Could you check a few things on this model? Use its own coordinates, in mm. Face numbers are marked on the shaded views. Coordinates: 2 decimals unless noted, no trailing zeros. Loops run counter-clockwise (first coordinate to the right, second up) from the corner with the lowest first, then second, coordinate; pieces in that order, holes last. Notation, with made-up numbers: (-18, -10) - (1, -10) arc R37 ccw to (1, 26) - close; hole circle Ø11 at (20, 24.25). An arc over 180 degrees is marked (long way). Use CSV: the item, a comma, the result in double quotes.
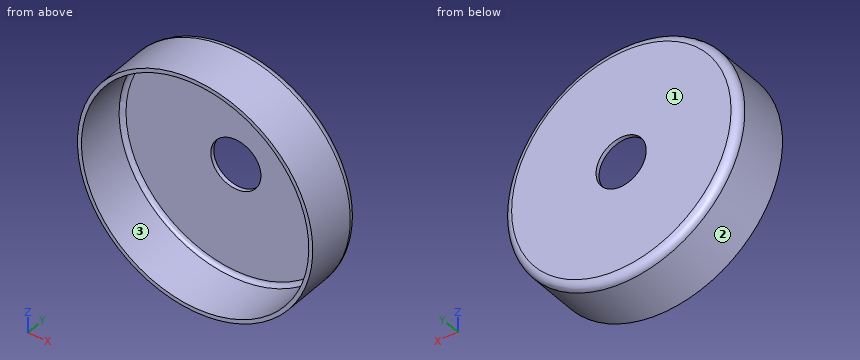
from build123d import *

# Parameters (mm, degrees)
SKETCH1_W               = 141.4859375
SKETCH1_H               = 69.85
FILLET1_R               = 9.525
SHELL1_T                = -4.7625
SKETCH3_R               = 30.1625
CUT_EXTRUDE1_DEPTH      = 30.734
CUT_EXTRUDE1_DEPTH_BACK = 28.194


with BuildPart() as part:
    # Sketch1 → Revolve1 (revolve)
    with BuildSketch(Plane(origin=(0, 0, 0), x_dir=(0, 0, -1), z_dir=(1, 0, 0)), mode=Mode.PRIVATE) as revolve1_sk:
        with Locations((-70.74296875, 34.925)):
            Rectangle(SKETCH1_W, SKETCH1_H)
    revolve(revolve1_sk.sketch.rotate(Axis((0, 0, 0), (0, 1, 0)), 180), axis=Axis((0, 0, 0), (0, 1, 0)))

    # Fillet1
    fillet1_edges = [part.edges().sort_by_distance(p)[0] for p in [
        (0, 69.85, 141.4859375),
    ]]
    fillet(fillet1_edges, radius=FILLET1_R)

    # Shell1
    shell1_openings = [part.faces().sort_by_distance(p)[0] for p in [
        (0, 0, 0),
    ]]
    offset(amount=SHELL1_T, openings=shell1_openings, kind=Kind.INTERSECTION)

    # Sketch3 → Cut-Extrude1 (cut, two sides)
    with BuildSketch(Plane(origin=(0, 69.85, 0), x_dir=(1, 0, 0), z_dir=(0, 1, 0))) as cut_extrude1_sk:
        with Locations(Location((0.218944766, 1.810655032, 0), (0, 0, 90))):
            Circle(SKETCH3_R)
    extrude(amount=CUT_EXTRUDE1_DEPTH, mode=Mode.SUBTRACT)
    extrude(cut_extrude1_sk.sketch, amount=-CUT_EXTRUDE1_DEPTH_BACK, mode=Mode.SUBTRACT)


solid = part.part
(1) Will these pins go through, and if not, where does the flat tip stop? pin 1 (3 mm diameter, centred on x = 36, y = 53.5, fed in from +Z); pin 2 (5 mm diameter, centred on x = 17, z = -28, fed in from -Y); pin 3 (8 mm diameter, centred on y = 42, z = -88.5, fed in from +X).
Computed:
pin 1,"stops at z = 137.22"
pin 2,"stops at y = 65.09"
pin 3,"stops at x = 113.48"
(2) Please list where these lines run through material, in increasing order: line 1 (X direction, y = 32, z = 0); line 2 (Y direction, x = -46.5, z = -72.5); line 3 (X direction, y = 21, z = 107.5).
Computed:
line 1,"x = -141.49 to -136.72, 136.72 to 141.49"
line 2,"y = 65.09 to 69.85"
line 3,"x = -91.99 to -84.48, 84.48 to 91.99"
(3) Thinking about a two-plate mould opening in X: for the marked faces 1, 2 and 3, which applies, +X half, -X half, draft (parallel to the pull), parting line (faces both ways), or undercut?
Computed:
face 1,"draft"
face 2,"parting line"
face 3,"undercut"
(4) Suppose I cut it at B-B (y = 44). Write out the boundary of the cut face in (x, z).
Computed:
outline,"circle Ø282.97 at (0, 0); hole circle Ø273.45 at (0, 0)"
